```python
from build123d import *

# Parameters (mm, degrees)
SKETCH1_R           = 4.7625
BOSS_EXTRUDE1_DEPTH = 6.604
CUT_EXTRUDE1_DEPTH  = 7.604
SKETCH3_W           = 6.604
SKETCH3_H           = 6.35
BOSS_EXTRUDE2_DEPTH = 6.604
FILLET1_R           = 6.35
FILLET2_R           = 3.175


with BuildPart() as part:
    # Sketch1 → Boss-Extrude1 (new body)
    with BuildSketch(Plane.XY):
        Polygon((0, 0), (0, 47.625), (-6.35, 47.625), (-6.35, 69.85), (-37.719, 69.85), (-37.719, 50.8), (-25.4, 38.481), (-25.4, 0), align=None)
        with Locations((-27.7495, 57.15)):
            Circle(SKETCH1_R, mode=Mode.SUBTRACT)
    extrude(amount=BOSS_EXTRUDE1_DEPTH)

    # Sketch2 → Cut-Extrude1 (cut, through all)
    with BuildSketch(Plane.XY.offset(6.604)):
        Polygon((-12.2936, 37.0078), (-13.716, 37.0078), (-13.716, 32.8422), (-12.2936, 32.8422), (-12.2936, 30.5562), (-6.35, 30.5562), (-6.35, 32.8422), (0, 32.8422), (0, 37.0078), (-6.35, 37.0078), (-6.35, 39.2938), (-12.2936, 39.2938), align=None)
        Polygon((-12.2936, 20.2438), (-12.2936, 17.9578), (-13.716, 17.9578), (-13.716, 13.7922), (-12.2936, 13.7922), (-12.2936, 11.5062), (-6.35, 11.5062), (-6.35, 13.7922), (0, 13.7922), (0, 17.9578), (-6.35, 17.9578), (-6.35, 20.2438), align=None)
    extrude(amount=-CUT_EXTRUDE1_DEPTH, mode=Mode.SUBTRACT)

    # Sketch3 → Boss-Extrude2 (add)
    with BuildSketch(Plane.XY.offset(6.604)):
        with Locations((3.302, 44.45)):
            Rectangle(SKETCH3_W, SKETCH3_H)
        with Locations((3.302, 25.4)):
            Rectangle(SKETCH3_W, SKETCH3_H)
        with Locations((3.302, 6.35)):
            Rectangle(SKETCH3_W, SKETCH3_H)
    extrude(amount=-BOSS_EXTRUDE2_DEPTH)

    # Fillet1
    fillet1_edges = [part.edges().sort_by_distance(p)[0] for p in [
        (-25.4, 0, 3.302),
        (-25.4, 38.481, 3.302),
        (-37.719, 50.8, 3.302),
        (-6.35, 69.85, 3.302),
        (-6.35, 47.625, 3.302),
    ]]
    fillet(fillet1_edges, radius=FILLET1_R)

    # Fillet2
    fillet2_edges = [part.edges().sort_by_distance(p)[0] for p in [
        (-37.719, 69.85, 3.302),
    ]]
    fillet(fillet2_edges, radius=FILLET2_R)


solid = part.part
```
Work out the finished part from the listing and answer in its coordinate system (mm). A direction names the side the tool comes from. Coordinates: 2 decimals unless noted, no trailing zeros. Loops run counter-clockwise (first coordinate to the right, second up) from the corner with the lowest first, then second, coordinate; pieces in that order, holes last. Notation, with made-up numbers: (77, 21.25) -> (97, 21.25) arc R18 ccw to (97, 26.25) -> close; hole circle Ø10 at (-15, 67). An arc over 180 degrees is marked (long way). Answer as CSV lines item,"result".
Q1. For a pull along Y with two mould halves and no side action, classify faces 1 (the face through (6.604, 44, 3)), 2 (the face through (3, 47.625, 3)), 3 (the face through (-3, 17.958, 3)) as +Y half, -Y half, draft (parallel to the pull), parting line (faces both ways), or undercut.
Findings:
face 1,"draft"
face 2,"+Y half"
face 3,"undercut"
Q2. The part is cut by section A-A on y = 57.15. Write down the section's boundary in (x, z), and give its area (3 significant figures).
Findings:
outline,"(-37.72, 0) -> (-32.51, 0) -> (-32.51, 6.6) -> (-37.72, 6.6) -> close; (-22.99, 0) -> (-6.35, 0) -> (-6.35, 6.6) -> (-22.99, 6.6) -> close"
area,"144 mm²"
Q3. Each of these flat-tipped pins is pushed along its axis until it touches: pin 1 (2.5 mm diameter, centred on y = 12.5, z = 2.5, fed in from +X); pin 2 (1.1 mm diameter, centred on y = 12.5, z = 2.5, fed in from -X); pin 3 (2 mm diameter, centred on y = 15.5, z = 2, fed in from +X). Where does it stop, or does it pass through?
Findings:
pin 1,"stops at x = 0"
pin 2,"stops at x = -25.4"
pin 3,"stops at x = -13.72"
Q4. Find the intervals of material crossed by probe 1 along Y at (x, z) = (-13.5, 2); probe 2 along Y at (x, z) = (1.5, 5.5) (3 decimals); probe 3 along X at (y, z) = (20, 2.5), in increasing order.
Findings:
probe 1,"y = 0 to 13.79, 17.96 to 32.84, 37.01 to 69.85"
probe 2,"y = 3.175 to 9.525, 22.225 to 28.575, 41.275 to 47.625"
probe 3,"x = -25.4 to -12.29, -6.35 to 0"
Q5. A tool of negligible diameter and unlimited length cuts with its end or side. For faces 4 (the face through (0, 20, 3)), 5 (the face through (-25.4, 21, 3)), 6 (the face through (-4.539, 49.535, 3.348)), 7 (the face through (-12.294, 32, 3)), from which of +Z, -Z, +X, -X, +Y, -Y can it reach the whole face along a straight path? Write none if from no direction.
Findings:
face 4,"+Z, -Z, +X"
face 5,"+Z, -Z, -X, -Y"
face 6,"+Z, -Z, +X, +Y"
face 7,"+Z, -Z"
